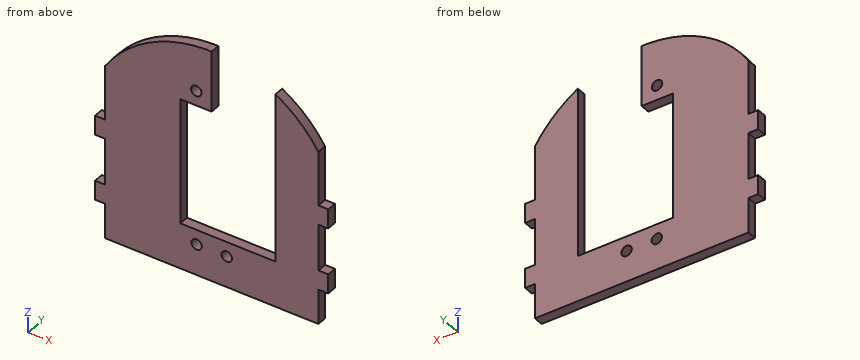
```python
from build123d import *

# Parameters (mm, degrees)
SKETCH1_W              = 70.104
SKETCH1_H              = 50.8
RECTANGULAR_BASE_DEPTH = 3.175
SKETCH4_W              = 3.2258
SKETCH4_H              = 6.35
TAB_DEPTH              = 3.175
SKETCH8_W              = 70.104
SKETCH8_H              = 25.4
BOSS_EXTRUDE2_DEPTH    = 3.175
CUT_EXTRUDE2_OUTLINE_R = 1.7145
CUT_EXTRUDE2_OUTLINE_W = 20.586
CUT_EXTRUDE2_OUTLINE_H = 41.275
CUT_EXTRUDE2_DEPTH     = 3.175
CUT_EXTRUDE3_DEPTH     = 64.686031419
CUT_EXTRUDE4_DEPTH     = 64.686031419


# Read off the part's stored shape, not the designer's step: Cut-Extrude2
with BuildPart() as part:
    # Sketch1 → rectangular base (new body)
    with BuildSketch(Plane(origin=(0, 0, 0), x_dir=(1, 0, 0), z_dir=(0, 1, 0))):
        Rectangle(SKETCH1_W, SKETCH1_H)
    extrude(amount=RECTANGULAR_BASE_DEPTH)

    # Sketch4 → tab (add)
    with BuildSketch(Plane(origin=(0, 3.175, 0), x_dir=(1, 0, 0), z_dir=(0, 1, 0))):
        with Locations((-36.6649, 10.795)):
            Rectangle(SKETCH4_W, SKETCH4_H)
        with Locations((-36.6649, -10.795)):
            Rectangle(SKETCH4_W, SKETCH4_H)
    tab = extrude(amount=-TAB_DEPTH)

    # Mirror1: tab across plane
    add(tab.mirror(Plane(origin=(0, 0, 0), x_dir=(0, 0, 1), z_dir=(1, 0, 0))))

    # Sketch8 → Boss-Extrude2 (add)
    with BuildSketch(Plane(origin=(0, 3.175, 0), x_dir=(1, 0, 0), z_dir=(0, 1, 0))):
        with Locations((0, -38.1)):
            Rectangle(SKETCH8_W, SKETCH8_H)
    extrude(amount=-BOSS_EXTRUDE2_DEPTH)

    # Cut-Extrude2 outline → Cut-Extrude2 (cut)
    with BuildSketch(Plane(origin=(0, 0, 0), x_dir=(1, 0, 0), z_dir=(0, 1, 0))):
        with Locations((4.955, 15.24)):
            Circle(CUT_EXTRUDE2_OUTLINE_R)
        with Locations((-4.955, 15.24)):
            Circle(CUT_EXTRUDE2_OUTLINE_R)
        with Locations((4.853793359, -35.687)):
            Circle(CUT_EXTRUDE2_OUTLINE_R)
        with Locations((-5.056206641, -35.687)):
            Circle(CUT_EXTRUDE2_OUTLINE_R)
        with Locations((0, -10.2235)):
            Rectangle(CUT_EXTRUDE2_OUTLINE_W, CUT_EXTRUDE2_OUTLINE_H)
    extrude(amount=CUT_EXTRUDE2_DEPTH, mode=Mode.SUBTRACT)

    # Sketch9 → Cut-Extrude3 (cut, through all)
    with BuildSketch(Plane(origin=(0, 3.175, 0), x_dir=(1, 0, 0), z_dir=(0, 1, 0))):
        Polygon((0, -30.861), (0, -50.8), (10.293, -50.8), (20.961, -50.8), (20.961, 10.414), (10.293, 10.414), (10.293, -30.861), align=None)
    extrude(amount=-CUT_EXTRUDE3_DEPTH, mode=Mode.SUBTRACT)

    # Sketch10 → Cut-Extrude4 (cut, through all)
    with BuildSketch(Plane(origin=(0, 3.175, 0), x_dir=(1, 0, 0), z_dir=(0, 1, 0))):
        with BuildLine():
            Line((-35.052, -31.75), (-35.052, -60.151970588))
            Line((-35.052, -60.151970588), (35.052, -60.151970588))
            Line((35.052, -60.151970588), (35.052, -31.75))
            ThreePointArc((35.052, -31.75), (0, -50.84891964), (-35.052, -31.75))
        make_face()
    extrude(amount=-CUT_EXTRUDE4_DEPTH, mode=Mode.SUBTRACT)


solid = part.part
```
Model file for the job. Use its own axes, mm. Round coordinates to 2 decimals unless told otherwise and drop trailing zeros. Write each loop counter-clockwise with the first axis right and the second up, starting at its lowest first coordinate (ties: lowest second). Pieces come first, ordered by that corner, then holes. Notation, with made-up numbers: (16, 9) - (24, 9) arc R33 cw to (24, 47) - close; hole circle Ø9 at (41.5, 69.5). An arc over 180 degrees is marked (long way). One line per item, written item: value.
(1) Cut at A-A, the plane z = -15.24. Give the cut face in (x, y) (1 decimal), plus the area to 3 significant figures.
Values follow:
outline: (-35.1, 0) - (-6.7, 0) - (-6.7, 3.2) - (-35.1, 3.2) - close; (-3.2, 0) - (3.2, 0) - (3.2, 3.2) - (-3.2, 3.2) - close; (6.7, 0) - (35.1, 0) - (35.1, 3.2) - (6.7, 3.2) - close
area: 201 mm²
(2) Cut at D-D, the plane x = 9. Give the cut face in (y, z) (3 decimals), plus the area to 3 significant figures.
Values follow:
outline: (0, -25.4) - (3.175, -25.4) - (3.175, -10.414) - (0, -10.414) - close
area: 47.6 mm²
(3) Wall check: probe 1 along X at (y, z) = (2.35, -15.24); probe 2 along X at (y, z) = (0.6, 18.5); probe 3 along X at (y, z) = (2.05, 35.5). Give the ranges that are in metal, low to high.
Values follow:
probe 1: x = -35.05 to -6.67, -3.24 to 3.24, 6.67 to 35.05
probe 2: x = -35.05 to -10.29, 20.96 to 35.05
probe 3: x = -32.33 to -6.76, -3.35 to 0, 20.96 to 32.33
(4) Cut at C-C, the plane y = 0.5. Give the number of separate pieces and of enclosed holes in the cut face, plus the area to 3 significant figures.
Values follow:
separate pieces: 1
enclosed holes: 3
area: 3,330 mm²
(5) Drop flat-ended pins along their axis: P1, Ø1.6, axis at y = 1, z = 16.5, coming from the +X side; P2, Ø1, axis at x = -36.5, y = 1, coming from the +Z side; P3, Ø1, axis at x = 16.5, y = 0.5, coming from the +Z side. Give the stop position or say it passes through.
Values follow:
P1: stops at x = 35.05
P2: stops at z = 13.97
P3: stops at z = -10.41
(6) Cut at B-B, the plane z = 2. Give the cut face in (x, y) (3 decimals), plus the area to 3 significant figures.
Values follow:
outline: (-35.052, 0) - (-10.293, 0) - (-10.293, 3.175) - (-35.052, 3.175) - close; (20.961, 0) - (35.052, 0) - (35.052, 3.175) - (20.961, 3.175) - close
area: 123 mm²
